from build123d import *

# Parameters (mm, degrees)
CUT_EXTRUDE2_DEPTH      = 40.744307769
CUT_EXTRUDE2_DEPTH_BACK = 40.744307769
SKETCH4_W               = 25.011127608
SKETCH4_H               = 6
CUT_EXTRUDE3_DEPTH      = 40.744307905
CUT_EXTRUDE3_DEPTH_BACK = 40.744307905
SKETCH3_4_R             = 2.5
CUT_EXTRUDE4_DEPTH      = 40.744307905
CUT_EXTRUDE4_DEPTH_BACK = 6


with BuildPart() as part:
    # Sketch2 → Revolve1 (revolve)
    with BuildSketch(Plane(origin=(0, 0, 0), x_dir=(0, 0, -1), z_dir=(1, 0, 0)), mode=Mode.PRIVATE) as revolve1_sk:
        Polygon((-33.1, 4), (0, 4), (0, 3), (20, 3), (20, 8), (-38.1, 8), (-38.1, 6), (-33.1, 6), align=None)
    revolve(revolve1_sk.sketch.rotate(Axis((0, 0, 12.975169934), (0, 0, -1)), 90), axis=Axis((0, 0, 12.975169934), (0, 0, -1)))

    # Sketch3 → Cut-Extrude2 (cut, two sides)
    with BuildSketch(Plane(origin=(0, 0, 0), x_dir=(1, 0, 0), z_dir=(0, 1, 0))) as cut_extrude2_sk:
        with BuildLine():
            Line((8, 0), (8, 25))
            Line((8, 25), (-8, 25))
            Line((-8, 25), (-8, 0))
            Line((-8, 0), (-3.753065966, 11.519523043))
            ThreePointArc((-3.753065966, 11.519523043), (0, 14.13586996), (3.753065966, 11.519523043))
            Line((3.753065966, 11.519523043), (8, 0))
        make_face()
    extrude(amount=CUT_EXTRUDE2_DEPTH, mode=Mode.SUBTRACT)
    extrude(cut_extrude2_sk.sketch, amount=-CUT_EXTRUDE2_DEPTH_BACK, mode=Mode.SUBTRACT)

    # Sketch4 → Cut-Extrude3 (cut, two sides)
    with BuildSketch(Plane(origin=(0, 0, 0), x_dir=(0, 0, -1), z_dir=(1, 0, 0))) as cut_extrude3_sk:
        with Locations((12.505563804, 0)):
            Rectangle(SKETCH4_W, SKETCH4_H)
    extrude(amount=CUT_EXTRUDE3_DEPTH, mode=Mode.SUBTRACT)
    extrude(cut_extrude3_sk.sketch, amount=-CUT_EXTRUDE3_DEPTH_BACK, mode=Mode.SUBTRACT)

    # Sketch3<4> → Cut-Extrude4 (cut, two sides)
    with BuildSketch(Plane(origin=(0, 0, 0), x_dir=(1, 0, 0), z_dir=(0, 1, 0))) as cut_extrude4_sk:
        with Locations(Location((0, 10.13586996, 0), (0, 0, 270))):
            Circle(SKETCH3_4_R)
    extrude(amount=CUT_EXTRUDE4_DEPTH, mode=Mode.SUBTRACT)
    extrude(cut_extrude4_sk.sketch, amount=-CUT_EXTRUDE4_DEPTH_BACK, mode=Mode.SUBTRACT)


solid = part.part
Design review of the part built by this model. Coordinates are the model's own, in mm. A direction names the side the tool comes from. Give positions to 0.01 mm unless a question says otherwise; leave off trailing zeros. Loops run counter-clockwise (first coordinate to the right, second up) from the corner with the lowest first, then second, coordinate; pieces in that order, holes last. Notation, with made-up numbers: M 5,78 L 21,78 A24 ccw 21,107 Z; hole C 44,-18.75 d1. An arc over 180 degrees is marked long. Write item = value, one per line.
Q1. We need section B-B (x = 0). Give the boundary of the cut face in (y, z).
Output values:
outline = M -8,-14.14 L -3,-14.14 L -3,-12.64 L -6,-12.64 L -6,-7.64 L -3,-7.64 L -3,0 L -4,0 L -4,33.1 L -6,33.1 L -6,38.1 L -8,38.1 Z; M 3,-14.14 L 8,-14.14 L 8,-12.64 L 3,-12.64 Z; M 3,-7.64 L 8,-7.64 L 8,38.1 L 6,38.1 L 6,33.1 L 4,33.1 L 4,0 L 3,0 Z
Q2. We need section A-A (y = 0). Give the boundary of the cut face in (x, z), plus the area to 3 significant figures.
Output values:
outline = M -8,0 L -4,0 L -4,33.1 L -6,33.1 L -6,38.1 L -8,38.1 Z; M 4,0 L 8,0 L 8,38.1 L 6,38.1 L 6,33.1 L 4,33.1 Z
area = 285 mm^2
Q3. For faces 4 (the flat face through (-5.2, -4.6, -7.6)), 5 (the flat face through (5.15, -4.55, -7.73)), 6 (the cylindrical face through (0.11, -4.479, -12.633)), 7 (the flat face through (0, -3.4, 0)), 8 (the flat face through (-6, 0, 0)), list the 3-axis set-ups (+Z, -Z, +X, -X, +Y, -Y) from which the entire face can be reached by the end or side of a thin tool; tool diameter is ignored.
Output values:
face_4 = -Z, -X, +Y, -Y
face_5 = -Z, +X, +Y, -Y
face_6 = +Y
face_7 = +Z
face_8 = -Z, +X, -X
Q4. We need section C-C (z = -1). Give the boundary of the cut face in (x, y), plus the area to 3 significant figures.
Output values:
outline = M -7.42,-3 A8 ccw 7.42,-3 Z; M -7.42,3 L 7.42,3 A8 ccw Z
area = 107 mm^2
Q5. To check wall thickness, follow line 1 (Y direction, x = 0, z = 35.95); line 2 (Z direction, x = 0, y = 5.25); line 3 (Z direction, x = -6.5, y = 0.5). State the ranges of each line that lie inside material, in increasing order. Write a range as [from, to].
Output values:
line_1 = [-8, -6], [6, 8]
line_2 = [-14.14, -12.64], [-7.64, 33.1]
line_3 = [0, 38.1]
Q6. We need section D-D (x = -3.25). Give the boundary of the cut face in (y, z).
Output values:
outline = M -7.31,-12.47 L -3,-12.47 L -3,0 L -2.33,0 L -2.33,33.1 L -5.04,33.1 L -5.04,38.1 L -7.31,38.1 Z; M 2.33,0 L 3,0 L 3,-12.47 L 7.31,-12.47 L 7.31,38.1 L 5.04,38.1 L 5.04,33.1 L 2.33,33.1 Z
Q7. Draft analysis for pull direction Y (two halves, no side actions). For faces 1 (the cylindrical face through (2.48, 5.47, -10.46)), 2 (the flat face through (6, 0, 0)), 3 (the cylindrical face through (4.301, -6.746, 18.152)), state which applies: +Y half, -Y half, draft (parallel to the pull), parting line (faces both ways), or undercut.
Output values:
face_1 = draft
face_2 = undercut
face_3 = parting line
Q8. Insertion check: pin 1 (4 mm diameter, centred on y = -6, z = -2, fed in from -X); pin 2 (3 mm diameter, centred on x = -4, z = 19.5, fed in from -Y); pin 3 (0.8 mm diameter, centred on x = -1, y = 3.5, fed in from +Z). Each pin has a flat end and moves straight along its axis. Give the tip position at first contact, or say it passes through.
Output values:
pin_1 = -6.93
pin_2 = -7.6
pin_3 = 33.1
